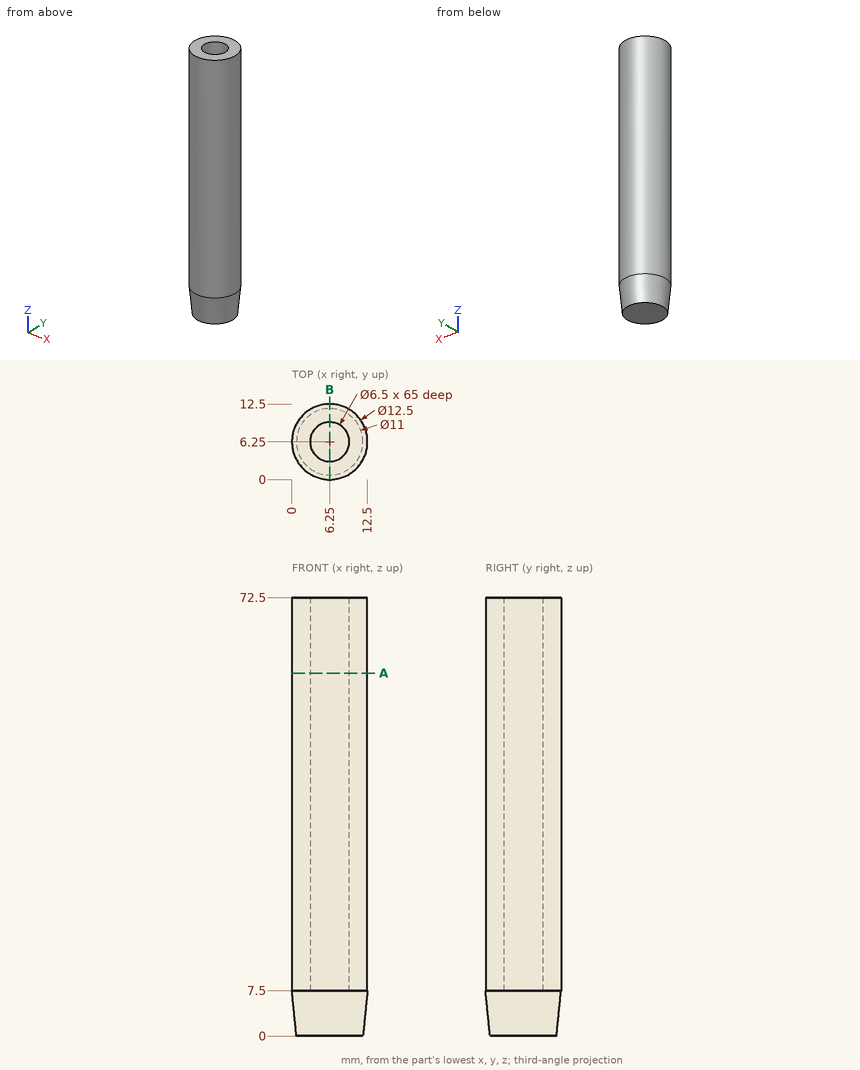
Study the drawing (mm; zero at the part's minimum x, y, z) and answer. Round coordinates to 2 decimals unless told otherwise and drop trailing zeros. Order: outer loops, then holes, each group sorted by start corner. A loop starts at its lowest first (then second) coordinate and runs counter-clockwise, first axis right, second up. Notation, with made-up numbers: (-21.75, 42.25) -> (36.25, 42.25) arc R14 cw to (36.25, 65.25) -> close; hole circle Ø8 at (-35, -17). An arc over 180 degrees is marked (long way). Answer as CSV lines item,"result". Start each with the question number.
(1) Find the intervals of material crossed by probe 1 along Y at (x, z) = (6.25, 26.5); probe 2 along Z at (x, y) = (7.5, 7.75); probe 3 along X at (y, z) = (4.25, 52), in increasing order. Write a range as from..to.
(2) The part is cut by section A-A (z = 60). Determine the outline of the cut face in (x, y).
(3) Flat-ended cylindrical pins translate along their axes: pin 1 Ø6 at (x, z) = (6, 35.5) entering from +Y; pin 2 Ø3 at (x, z) = (3, 41) entering from -Y; pin 3 Ø6 at (x, y) = (6.25, 6.25) entering from +Z; pin 4 Ø1.5 at (x, z) = (8, 17) entering from +Y. Find the tip coordinate at first contact, or state that the pin passes through.
(4) The part is cut by section B-B (x = 6.25). Determine the outline of the cut face in (y, z).
Evaluation:
1,probe 1,"0..3, 9.5..12.5"
1,probe 2,"0..7.5"
1,probe 3,"0.33..3.69, 8.81..12.17"
2,outline,"circle Ø12.5 at (6.25, 6.25); hole circle Ø6.5 at (6.25, 6.25)"
3,pin 1,"y = 12.5"
3,pin 2,"y = 0.25"
3,pin 3,"z = 7.5"
3,pin 4,"y = 12.42"
4,outline,"(0, 7.5) -> (0.75, 0) -> (11.75, 0) -> (12.5, 7.5) -> (12.5, 72.5) -> (9.5, 72.5) -> (9.5, 7.5) -> (3, 7.5) -> (3, 72.5) -> (0, 72.5) -> close"
